Verification items for the finished model (mm, model axes). A direction names the side the tool comes from. Coordinates: 2 decimals unless noted, no trailing zeros. Write each loop counter-clockwise with the first axis right and the second up, starting at its lowest first coordinate (ties: lowest second). Pieces come first, ordered by that corner, then holes. Notation, with made-up numbers: (61, 72) -> (106, 72) arc R14 ccw to (106, 85) -> close; hole circle Ø8 at (-4.5, 52). An arc over 180 degrees is marked (long way). Answer in a Markdown table with one row per item.
```python
from build123d import *

# Parameters (mm, degrees)
SKETCH1_R           = 4.6
SKETCH1_R_2         = 2.5
BOSS_EXTRUDE1_DEPTH = 19
SKETCH1_3_R         = 4.6
SKETCH1_3_R_2       = 2.5
SKETCH1_3_R_3       = 2
BOSS_EXTRUDE2_DEPTH = 1.6
SKETCH1_4_R         = 2
BOSS_EXTRUDE3_DEPTH = 0.8
SKETCH1_5_R         = 2.5
BOSS_EXTRUDE4_DEPTH = 4
BOSS_EXTRUDE5_DEPTH = 6
FILLET1_R           = 1
FILLET2_R           = 1


with BuildPart() as part:
    # Sketch1 → Boss-Extrude1 (new body)
    # profile 1 of 3: a face of its own
    with BuildSketch(Plane(origin=(0, 0, 0), x_dir=(1, 0, 0), z_dir=(0, 1, 0))):
        with BuildLine():
            ThreePointArc((11.466935703, 8.771283954), (-14.436938211, 0.029184365), (11.431379714, -8.817573048))
            Line((11.431379714, -8.817573048), (13.700622891, -8.817573048))
            Line((13.700622891, -8.817573048), (14.138880413, -7.25))
            Line((14.138880413, -7.25), (16.593765248, -7.25))
            Line((16.593765248, -7.25), (16.593765248, 7.25))
            Line((16.593765248, 7.25), (14.905644331, 7.25))
            Line((14.905644331, 7.25), (14.326809253, 8.771283954))
            Line((14.326809253, 8.771283954), (11.466935703, 8.771283954))
        make_face()
        with Locations((-8.506234752, 0)):
            Circle(SKETCH1_R, mode=Mode.SUBTRACT)
    # profile 2 of 3: a face of its own
    with BuildSketch(Plane(origin=(0, 0, 0), x_dir=(1, 0, 0), z_dir=(0, 1, 0))):
        with Locations((-8.506234752, 0)):
            Circle(SKETCH1_R)
        with Locations((-8.506234752, 0)):
            Circle(SKETCH1_R_2, mode=Mode.SUBTRACT)
    # profile 3 of 3: a face of its own
    with BuildSketch(Plane(origin=(0, 0, 0), x_dir=(1, 0, 0), z_dir=(0, 1, 0))):
        with Locations((-8.506234752, 0)):
            Circle(SKETCH1_R_2)
    extrude(amount=BOSS_EXTRUDE1_DEPTH)

    # Sketch1<3> → Boss-Extrude2 (add)
    # profile 1 of 2: a face of its own
    with BuildSketch(Plane(origin=(0, 0, 0), x_dir=(1, 0, 0), z_dir=(0, 1, 0))):
        with Locations(Location((-8.506234752, 0, 0), (0, 0, 270))):
            Circle(SKETCH1_3_R)
        with Locations(Location((-8.506234752, 0, 0), (0, 0, 270))):
            Circle(SKETCH1_3_R_2, mode=Mode.SUBTRACT)
    # profile 2 of 2: a face of its own
    with BuildSketch(Plane(origin=(0, 0, 0), x_dir=(1, 0, 0), z_dir=(0, 1, 0))):
        with Locations((-0.506234752, 17.5)):
            Circle(SKETCH1_3_R_3)
    extrude(amount=-BOSS_EXTRUDE2_DEPTH)


with BuildPart() as boss_extrude2_kept_piece:
    # of the separate pieces the step leaves, the one the design keeps (boss_extrude2_pieces_kept)
    add(part.part.solids().sort_by_distance((11.466935703, 0, -8.771283954))[0])

    # Sketch1<4> → Boss-Extrude3 (add)
    # profile 1 of 2: a face of its own
    with BuildSketch(Plane(origin=(0, 0, 0), x_dir=(1, 0, 0), z_dir=(0, 1, 0))):
        with BuildLine():
            ThreePointArc((-4.006234752, 13.869971872), (-0.52182238, 14.427534025), (2.993765248, 14.123151428))
            Line((2.993765248, 14.123151428), (2.993765248, 17.5))
            ThreePointArc((2.993765248, 17.5), (-0.506234752, 21), (-4.006234752, 17.5))
            Line((-4.006234752, 17.5), (-4.006234752, 13.869971872))
        make_face()
        with Locations(Location((-0.506234752, 17.5, 0), (0, 0, 270))):
            Circle(SKETCH1_4_R, mode=Mode.SUBTRACT)
    # profile 2 of 2: a face of its own
    with BuildSketch(Plane(origin=(0, 0, 0), x_dir=(1, 0, 0), z_dir=(0, 1, 0))):
        with BuildLine():
            ThreePointArc((2.993765248, -14.123151428), (-0.52182238, -14.427534025), (-4.006234752, -13.869971872))
            Line((-4.006234752, -13.869971872), (-4.006234752, -17.5))
            ThreePointArc((-4.006234752, -17.5), (-0.506234752, -21), (2.993765248, -17.5))
            Line((2.993765248, -17.5), (2.993765248, -14.123151428))
        make_face()
        with Locations(Location((-0.506234752, -17.5, 0), (0, 0, 270))):
            Circle(SKETCH1_4_R, mode=Mode.SUBTRACT)
    extrude(amount=BOSS_EXTRUDE3_DEPTH)

    # Sketch1<5> → Boss-Extrude4 (add)
    with BuildSketch(Plane(origin=(0, 0, 0), x_dir=(1, 0, 0), z_dir=(0, 1, 0))):
        with Locations(Location((-8.506234752, 0, 0), (0, 0, 270))):
            Circle(SKETCH1_5_R)
    extrude(amount=-BOSS_EXTRUDE4_DEPTH)

    # Sketch5 → Boss-Extrude5 (add)
    with BuildSketch(Plane.XZ.offset(4)):
        with BuildLine():
            Line((-9.968251002, 1.5), (-10.506234752, 1.5))
            ThreePointArc((-10.506234752, 1.5), (-11.006234752, 0), (-10.506234752, -1.5))
            Line((-10.506234752, -1.5), (-9.968251002, -1.5))
            Line((-9.968251002, -1.5), (-9.968251002, 1.5))
        make_face()
        with BuildLine():
            Line((-6.506234752, 1.5), (-9.968251002, 1.5))
            Line((-9.968251002, 1.5), (-9.968251002, -1.5))
            Line((-9.968251002, -1.5), (-6.506234752, -1.5))
            ThreePointArc((-6.506234752, -1.5), (-6.134526507, -0.790569415), (-6.006234752, 0))
            ThreePointArc((-6.006234752, 0), (-6.134526507, 0.790569415), (-6.506234752, 1.5))
        make_face()
    extrude(amount=BOSS_EXTRUDE5_DEPTH)

    # Fillet1
    # the kernel refuses this fillet: 1 mm, written as the material it adds along each edge
    with BuildSketch(Plane(origin=(-4.006234752, -4, 1.5), x_dir=(0, 0, 1), z_dir=(-1, 0, 0))) as fillet1_piece_1_section:
        with BuildLine():
            CenterArc((FILLET1_R, -FILLET1_R), FILLET1_R, 90, 90)
            Line((0, -FILLET1_R), (0, 0))
            Line((0, 0), (FILLET1_R, 0))
        make_face()
    fillet1_piece_1 = extrude(amount=9, mode=Mode.PRIVATE)
    fillet1_piece_1 = fillet1_piece_1 & Plane(origin=(-8.506234752, -4.243408623, 0), x_dir=(0, 0, 1), z_dir=(0, 1, 0)) * Cylinder(2.5, 22, mode=Mode.PRIVATE)
    add(fillet1_piece_1)

    # Fillet2
    # the kernel refuses this fillet: 1 mm, written as the material it adds along each edge
    with BuildSketch(Plane(origin=(-13.006234752, -4, -1.5), x_dir=(0, 0, -1), z_dir=(1, 0, 0))) as fillet2_piece_1_section:
        with BuildLine():
            CenterArc((FILLET2_R, -FILLET2_R), FILLET2_R, 90, 90)
            Line((0, -FILLET2_R), (0, 0))
            Line((0, 0), (FILLET2_R, 0))
        make_face()
    fillet2_piece_1 = extrude(amount=9, mode=Mode.PRIVATE)
    fillet2_piece_1 = fillet2_piece_1 & Plane(origin=(-8.506234752, -4.243408623, 0), x_dir=(0, 0, 1), z_dir=(0, 1, 0)) * Cylinder(2.5, 22, mode=Mode.PRIVATE)
    add(fillet2_piece_1)


solid = boss_extrude2_kept_piece.part
```
1. Sectioned sample at C-C, the plane z = 1. Record the cut outline in (x, y).
Findings below:
| item | result |
|---|---|
| outline | (-14.4, 0) -> (-13, 0) -> (-13, -1.6) -> (-10.8, -1.6) -> (-10.8, -10) -> (-6.21, -10) -> (-6.21, -1.6) -> (-4.02, -1.6) -> (-4.02, 0) -> (16.59, 0) -> (16.59, 19) -> (-14.4, 19) -> close |
2. Go/stop test with flat-tipped pins: pin 1 (4 mm diameter, centred on y = 1.5, z = -12.5, fed in from -X); pin 2 (1.5 mm diameter, centred on x = 11, y = 0, fed in from +Z); pin 3 (0.7 mm diameter, centred on x = 12, y = 10.5, fed in from +Z). Record where each tip stops, or that it passes through.
Findings below:
| item | result |
|---|---|
| pin 1 | stops at x = -9.91 |
| pin 2 | stops at z = 10.17 |
| pin 3 | stops at z = 8.82 |
3. Material ranges on probe 1 along X at (y, z) = (0.55, -17.5); probe 2 along Y at (x, z) = (-8, 10.5); probe 3 along Z at (x, y) = (15, 10.25), recorded low to high. Write a range as from..to.
Findings below:
| item | result |
|---|---|
| probe 1 | x = -4.01..-2.51, 1.49..2.99 |
| probe 2 | y = 0..19 |
| probe 3 | z = -7.25..7.25 |
4. Release check for a two-part mould opening along X. For faces 1 (the face through (13.92, 9.37, 8.04)), 2 (the face through (16, 9, -7.25)), 3 (the face through (-1.72, 0.39, -19.09)) record: released by +X, released by -X, zero draft, split by the parting line, or undercut.
Findings below:
| item | result |
|---|---|
| face 1 | released by +X |
| face 2 | zero draft |
| face 3 | undercut |
5. Sectioned sample at A-A, the plane x = -1.5. Record the cut outline in (y, z), and give its area (3 significant figures).
Findings below:
| item | result |
|---|---|
| outline | (0, -20.86) -> (0.8, -20.86) -> (0.8, -19.24) -> (0, -19.24) -> close; (0, -15.76) -> (0.8, -15.76) -> (0.8, -14.36) -> (19, -14.36) -> (19, 14.36) -> (0.8, 14.36) -> (0.8, 15.76) -> (0, 15.76) -> close; (0, 19.24) -> (0.8, 19.24) -> (0.8, 20.86) -> (0, 20.86) -> close |
| area | 550 mm² |
6. Access from +Z, -Z, +X, -X, +Y, -Y to the whole of each face (thin tool, end or side, straight path). Record for faces 4 (the face through (13, 9, -8.771)), 5 (the face through (-14.427, 9.367, -0.532)), 6 (the face through (-4.627, -0.789, 2.473)), 7 (the face through (13, 9, 8.818)), 8 (the face through (-8.5, -4.4, 1.7)).
Findings below:
| item | result |
|---|---|
| face 4 | -Z, +X, +Y, -Y |
| face 5 | +Y |
| face 6 | -Y |
| face 7 | +Z, +X, +Y, -Y |
| face 8 | +Z, +X, -X, -Y |
7. Sectioned sample at D-D, the plane x = -9.5. Record the cut outline in (y, z).
Findings below:
| item | result |
|---|---|
| outline | (-10, -1.5) -> (-5, -1.5) arc R1 cw to (-4.02, -2.29) -> (-1.6, -2.29) -> (-1.6, -4.49) -> (0, -4.49) -> (0, -10.87) -> (19, -10.87) -> (19, 10.87) -> (0, 10.87) -> (0, 4.49) -> (-1.6, 4.49) -> (-1.6, 2.29) -> (-4.02, 2.29) arc R1 cw to (-5, 1.5) -> (-10, 1.5) -> close |
8. Sectioned sample at B-B, the plane y = 14.75. Record the cut outline in (x, z), and give its area (3 significant figures).
Findings below:
| item | result |
|---|---|
| outline | (11.43, 8.82) arc R14.44 ccw (long way) to (11.47, -8.77) -> (14.33, -8.77) -> (14.91, -7.25) -> (16.59, -7.25) -> (16.59, 7.25) -> (14.14, 7.25) -> (13.7, 8.82) -> close |
| area | 702 mm² |
